Here's how the part is built. I have some questions about the finished solid (model axes, mm). Face numbers are marked on the shaded views. A direction names the side the tool comes from. Round coordinates to 2 decimals unless told otherwise and drop trailing zeros. Loops run counter-clockwise (first coordinate to the right, second up) from the corner with the lowest first, then second, coordinate; pieces in that order, holes last. Notation, with made-up numbers: (-25.75, -11.5) -> (16.25, -11.5) arc R32 cw to (16.25, 27.5) -> close; hole circle Ø11 at (47, -25). An arc over 180 degrees is marked (long way). One line per item, written item: value. Start each with the question number.
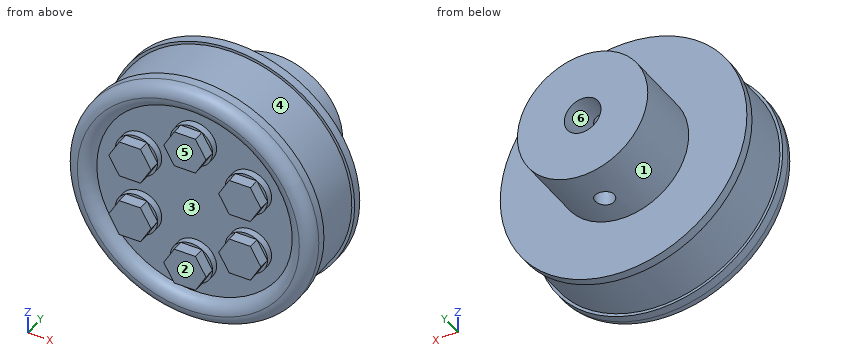
```python
from build123d import *

# Parameters (mm, degrees)
F0_R      = 22.225
F1_DEPTH  = 12.7
F2_R      = 3.81
F3_DEPTH  = 1.27
F5_DEPTH  = 2.032
F6_R      = 22.225
F6_R_2    = 17.78
F7_DEPTH  = 2.2225
F8_R      = 2.22249
F9_R      = 2.2225
F10_R     = 11.7475
F11_DEPTH = 12.7
F12_R     = 3.302
F13_DEPTH = 6.35
F14_R     = 1.7272
F15_DEPTH = 63.5
F16_W     = 9.525
F16_H     = 0.508


# Not quite as in the source:
# - a fillet or chamfer is up to 0.001 mm smaller than in the source, because OpenCascade refuses the exact size


with BuildPart() as f1:
    # F0 (on Front) → F1 (new body)
    with BuildSketch(Plane.XZ):
        Circle(F0_R)
    extrude(amount=F1_DEPTH)

    # F2 (on face) → F3 (join)
    with BuildSketch(Plane.XZ.offset(12.7)):
        with Locations((0, 11.43)):
            Circle(F2_R)
        with Locations((-9.8986703653, 5.715)):
            Circle(F2_R)
        with Locations((-9.8986703653, -5.715)):
            Circle(F2_R)
        with Locations((0, -11.43)):
            Circle(F2_R)
        with Locations((9.8986703653, -5.715)):
            Circle(F2_R)
        with Locations((9.8986703653, 5.715)):
            Circle(F2_R)
    extrude(amount=F3_DEPTH)

    # F4 (on face) → F5 (join)
    with BuildSketch(Plane.XZ.offset(13.97)):
        Polygon((1.905, 8.1304432116), (3.81, 11.43), (1.905, 14.7295567884), (-1.905, 14.7295567884), (-3.81, 11.43), (-1.905, 8.1304432116), align=None)
        Polygon((-7.9936703653, 2.4154432116), (-6.0886703653, 5.715), (-7.9936703653, 9.0145567884), (-11.8036703653, 9.0145567884), (-13.7086703653, 5.715), (-11.8036703653, 2.4154432116), align=None)
        Polygon((7.9936703653, 9.0145567884), (6.0886703653, 5.715), (7.9936703653, 2.4154432116), (11.8036703653, 2.4154432116), (13.7086703653, 5.715), (11.8036703653, 9.0145567884), align=None)
        Polygon((-7.9936703653, -2.4154432116), (-11.8036703653, -2.4154432116), (-13.7086703653, -5.715), (-11.8036703653, -9.0145567884), (-7.9936703653, -9.0145567884), (-6.0886703653, -5.715), align=None)
        Polygon((3.81, -11.43), (1.905, -8.1304432116), (-1.905, -8.1304432116), (-3.81, -11.43), (-1.905, -14.7295567884), (1.905, -14.7295567884), align=None)
        Polygon((7.9936703653, -2.4154432116), (6.0886703653, -5.715), (7.9936703653, -9.0145567884), (11.8036703653, -9.0145567884), (13.7086703653, -5.715), (11.8036703653, -2.4154432116), align=None)
    extrude(amount=F5_DEPTH)

    # F6 (on face) → F7 (join)
    with BuildSketch(Plane.XZ.offset(12.7)):
        Circle(F6_R)
        Circle(F6_R_2, mode=Mode.SUBTRACT)
    extrude(amount=F7_DEPTH)

    # F8 (radius 2.2225 in the source; OpenCascade refuses exactly that, so slightly less here)
    f8_edges = [f1.edges().sort_by_distance(p)[0] for p in [
        (-17.78, -14.9225, 0),
    ]]
    fillet(f8_edges, radius=F8_R)

    # F9
    f9_edges = [f1.edges().sort_by_distance(p)[0] for p in [
        (-22.225, -14.9225, 0),
    ]]
    fillet(f9_edges, radius=F9_R)

    # F10 (on face) → F11 (join)
    with BuildSketch(Plane(origin=(0, 0, 0), x_dir=(-1, 0, 0), z_dir=(0, 1, 0))):
        Circle(F10_R)
    extrude(amount=F11_DEPTH)

    # F12 (on face) → F13 (cut)
    with BuildSketch(Plane(origin=(0, 12.7, 0), x_dir=(-1, 0, 0), z_dir=(0, 1, 0))):
        Circle(F12_R)
    extrude(amount=-F13_DEPTH, mode=Mode.SUBTRACT)

    # F14 (on Top) → F15 (cut, symmetric)
    with BuildSketch(Plane.XY):
        with Locations((0, 5.842)):
            Circle(F14_R)
    extrude(amount=F15_DEPTH, both=True, mode=Mode.SUBTRACT)

    # F16 (on Right) → F18 (revolve, cut)
    with BuildSketch(Plane.YZ):
        with Locations((-6.35, 22.479)):
            Rectangle(F16_W, F16_H)
        with Locations((-6.35, 21.971)):
            Rectangle(F16_W, F16_H)
    revolve(axis=Axis((0, 11.6996625438, 0), (0, 1, 0)), mode=Mode.SUBTRACT)


solid = f1.part
```
Q1. If I drill on line 1 along Z through (x, y) = (0, 11.25); line 2 along Y through (x, z) = (3.5, -1); line 3 along Y through (x, z) = (10.5, -7), over which ranges is the centre line in solid material (lowest first)?
Q2. Which directions (+Z, -Z, +X, -X, +Y, -Y) give clear straight access to the entire face, cutting with the end or side of a thin tool? Please do the marked faces 4, 5 and 6.
Q3. I want a section at C-C on y = 8.25. Please give me the cut outline in (x, z) (1 decimal).
Q4. I want a section at B-B on y = -7.25. Please give me the cut outline in (x, z).
Q5. If we mould it in two halves opening along X, with no side actions, what happens to the marked faces 1, 2 and 3? For each: released by +X, released by -X, zero draft, split by the parting line, or undercut.
Q6. Will these pins go through, and if not, where does the flat tip stop? P1, Ø6, axis at x = 0, z = 0, coming from the +Y side; P2, Ø1, axis at x = -0.5, y = -14.5, coming from the +Z side; P3, Ø5, axis at y = 9, z = 10, coming from the +X side.
Answers below:
1. line 1: z = -11.75 to -3.3, 3.3 to 11.75
1. line 2: y = -12.7 to 12.7
1. line 3: y = -16 to 0
2. face 4: none
2. face 5: +Z, -Z, +X, -X, -Y
2. face 6: +Y
3. outline: circle Ø23.5 at (0, 0); hole circle Ø6.6 at (0, 0)
4. outline: circle Ø43.43 at (0, 0)
5. face 1: split by the parting line
5. face 2: zero draft
5. face 3: undercut
6. P1: stops at y = 6.35
6. P2: stops at z = 21.8
6. P3: stops at x = 9.04
